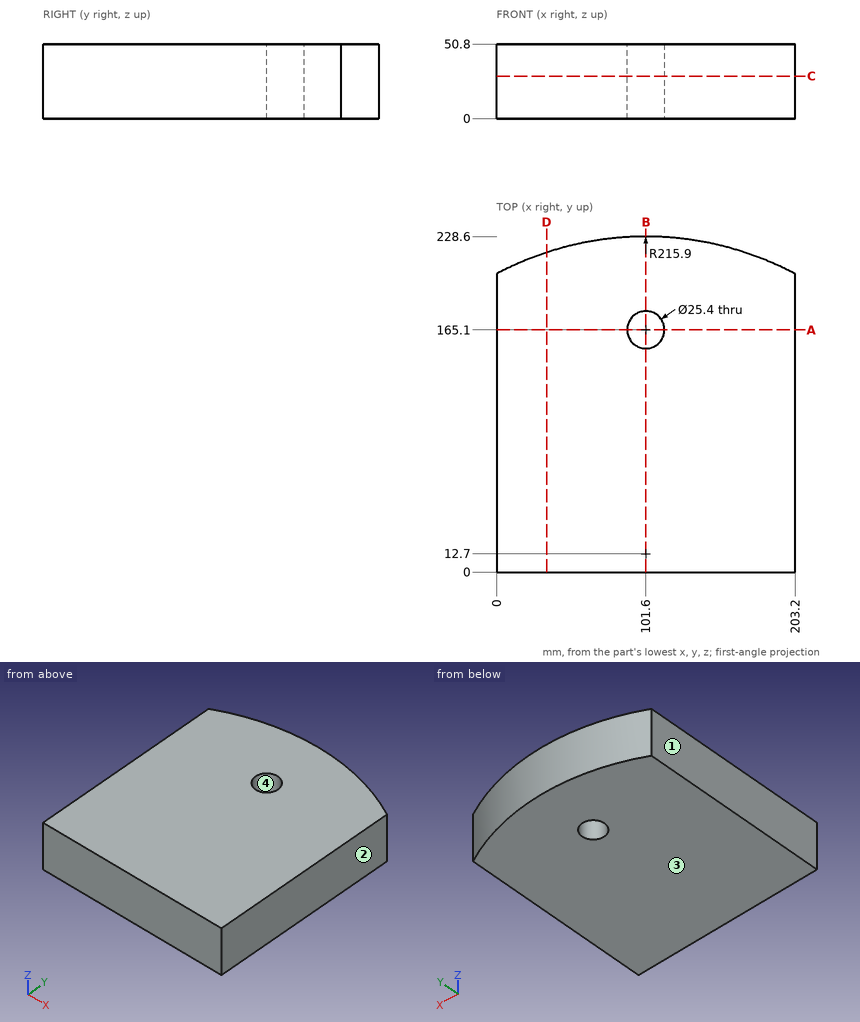
Verification items for this drawing (mm, ordinates from the low corner). Coordinates: 2 decimals unless noted, no trailing zeros. Loops run counter-clockwise (first coordinate to the right, second up) from the corner with the lowest first, then second, coordinate; pieces in that order, holes last. Notation, with made-up numbers: (16, 63) -> (67, 63) arc R29 cw to (67, 83) -> close; hole circle Ø3 at (82.5, 14.25). An arc over 180 degrees is marked (long way). Answer in a Markdown table with one row per item. Add a question column.
1. Draft check along X on the marked faces 1, 2, 3 and 4. Enter one of: +X half, -X half, draft (parallel to the pull), parting line (faces both ways), or undercut.
2. Section check C-C, the plane z = 29. Enter the section's corners in (x, y), then the cut area to 3 significant figures.
3. Depth check by flat-ended pin: P1, Ø20.5, axis at x = 101.6, y = 165.1, coming from the -Z side. Enter the tip coordinate at first touch or a pass-through.
4. Section check B-B, the plane x = 101.6. Enter the section's corners in (y, z).
5. Section check A-A, the plane y = 165.1. Enter the section's corners in (x, z).
6. Material ranges on probe 1 along X at (y, z) = (165, 37); probe 2 along X at (y, z) = (175, 13); probe 3 along Y at (x, z) = (101.6, 28), recorded low to high. Write a range as [from, to].
7. Section check D-D, the plane x = 34. Enter the section's corners in (y, z), then the cut area to 3 significant figures.
Derived:
| question | item | result |
|---|---|---|
| 1 | face 1 | -X half |
| 1 | face 2 | +X half |
| 1 | face 3 | draft |
| 1 | face 4 | undercut |
| 2 | outline | (0, 0) -> (203.2, 0) -> (203.2, 203.2) arc R215.9 ccw to (0, 203.2) -> close; hole circle Ø25.4 at (101.6, 165.1) |
| 2 | area | 44,300 mm² |
| 3 | P1 | passes through |
| 4 | outline | (0, 0) -> (152.4, 0) -> (152.4, 50.8) -> (0, 50.8) -> close; (177.8, 0) -> (228.6, 0) -> (228.6, 50.8) -> (177.8, 50.8) -> close |
| 5 | outline | (0, 0) -> (88.9, 0) -> (88.9, 50.8) -> (0, 50.8) -> close; (114.3, 0) -> (203.2, 0) -> (203.2, 50.8) -> (114.3, 50.8) -> close |
| 6 | probe 1 | x = [0, 88.9], [114.3, 203.2] |
| 6 | probe 2 | x = [0, 93.65], [109.55, 203.2] |
| 6 | probe 3 | y = [0, 152.4], [177.8, 228.6] |
| 7 | outline | (0, 0) -> (217.74, 0) -> (217.74, 50.8) -> (0, 50.8) -> close |
| 7 | area | 11,100 mm² |
